```python
from build123d import *

# Parameters (mm, degrees)
SKETCH_1_R      = 3
EXTRUDE_1_DEPTH = 1.6
CHAMFER_1_SIZE  = 1.6
SKETCH_2_R      = 1.4
EXTRUDE_2_DEPTH = 16.4
CHAMFER_2_SIZE  = 0.2


with BuildPart() as part:
    # 草图1 → 凸台-拉伸1 (new body)
    with BuildSketch(Plane(origin=(0, 0, 0), x_dir=(1, 0, 0), z_dir=(0, 1, 0))):
        with Locations(Location((0, 0, 0), (0, 0, 270))):
            Circle(SKETCH_1_R)
        Polygon((0, -1.154700538), (1, -0.577350269), (1, 0.577350269), (0, 1.154700538), (-1, 0.577350269), (-1, -0.577350269), align=None, mode=Mode.SUBTRACT)
    extrude(amount=EXTRUDE_1_DEPTH)

    # 倒角1
    # the kernel refuses this chamfer: 1.6 mm, written as the material it takes off along each edge
    with BuildSketch(Plane(origin=(0, 1.6, 0), x_dir=(0, 0, 1), z_dir=(-1, 0, 0))) as chamfer_1_piece_1:
        Polygon((3, -CHAMFER_1_SIZE), (3 - CHAMFER_1_SIZE, 0), (3, 0), align=None)
    revolve(axis=Axis((0, 1.6, 0), (0, 1, 0)), mode=Mode.SUBTRACT)

    # 草图2 → 凸台-拉伸2 (add)
    with BuildSketch(Plane(origin=(0, 1.6, 0), x_dir=(1, 0, 0), z_dir=(0, 1, 0))):
        with Locations(Location((0, 0, 0), (0, 0, 270))):
            Circle(SKETCH_2_R)
    extrude(amount=EXTRUDE_2_DEPTH)

    # 倒角2
    chamfer_2_edges = [part.edges().sort_by_distance(p)[0] for p in [
        (0, 18, -1.4),
    ]]
    chamfer(chamfer_2_edges, length=CHAMFER_2_SIZE)


solid = part.part
```
Geometry: final body of the model. Coordinates: model frame, mm. A direction names the side the tool comes from. Coordinates: 2 decimals unless noted, no trailing zeros. Order: outer loops, then holes, each group sorted by start corner. A loop starts at its lowest first (then second) coordinate and runs counter-clockwise, first axis right, second up. Notation, with made-up numbers: (66.5, 74.5) -> (83.5, 74.5) arc R20 cw to (83.5, 113.5) -> close; hole circle Ø2 at (15, 42). An arc over 180 degrees is marked (long way). Answer in a Markdown table with one row per item.
Item 1: Section A-A on z = 0. Output: boundary loops of the cut face in (x, y), plus the area to 3 significant figures.
Return value:
| item | result |
|---|---|
| outline | (-3, 0) -> (-1, 0) -> (-1, 1.6) -> (1, 1.6) -> (1, 0) -> (3, 0) -> (1.4, 1.6) -> (1.4, 17.8) -> (1.2, 18) -> (-1.2, 18) -> (-1.4, 17.8) -> (-1.4, 1.6) -> close |
| area | 49.7 mm² |
Item 2: Draft query along X for faces 1 (the flat face through (1, 1, 0)), 2 (the flat face through (0, 18, 0)), 3 (the cylindrical face through (0.06, 9.59, -1.4)). Return one class per face: released by +X, released by -X, zero draft, split by the parting line, or undercut.
Return value:
| item | result |
|---|---|
| face 1 | undercut |
| face 2 | zero draft |
| face 3 | split by the parting line |
Item 3: Contact query for flat-ended pins moving along their axis: P1, Ø0.6, axis at x = 0, z = 0, coming from the -Y side; P2, Ø2, axis at x = -2, y = 11.5, coming from the +Z side; P3, Ø1.3, axis at y = 1, z = 0, coming from the -X side. Output: stop coordinate, or through.
Return value:
| item | result |
|---|---|
| P1 | stops at y = 1.6 |
| P2 | stops at z = 0.98 |
| P3 | stops at x = -2.65 |
Item 4: Access query for faces 4 (the flat face through (-1.3, 0, 0)), 5 (the flat face through (0, 1.6, 0)). Directions: +Z, -Z, +X, -X, +Y, -Y. A direction counts if a zero-diameter tool reaches every point of the face in a straight line with its end or side. Return the directions, or none.
Return value:
| item | result |
|---|---|
| face 4 | +Z, -Z, +X, -X, -Y |
| face 5 | -Y |
Item 5: Ray query, L1, parallel to X at y = 12.5, z = 0.05; L2, parallel to Z at x = 0.5, y = 7.75. Return the intervals inside material, ascending.
Return value:
| item | result |
|---|---|
| L1 | x = -1.4 to 1.4 |
| L2 | z = -1.31 to 1.31 |
Item 6: Section B-B on y = 16.5. Output: boundary loops of the cut face in (x, z), plus the area to 3 significant figures.
Return value:
| item | result |
|---|---|
| outline | circle Ø2.8 at (0, 0) |
| area | 6.16 mm² |
